Could you check a few things on this drawing? It's one solid part, dimensions in mm from its lowest x, y, z. A direction names the side the tool comes from. Coordinates: 2 decimals unless noted, no trailing zeros. Write each loop counter-clockwise with the first axis right and the second up, starting at its lowest first coordinate (ties: lowest second). Pieces come first, ordered by that corner, then holes.
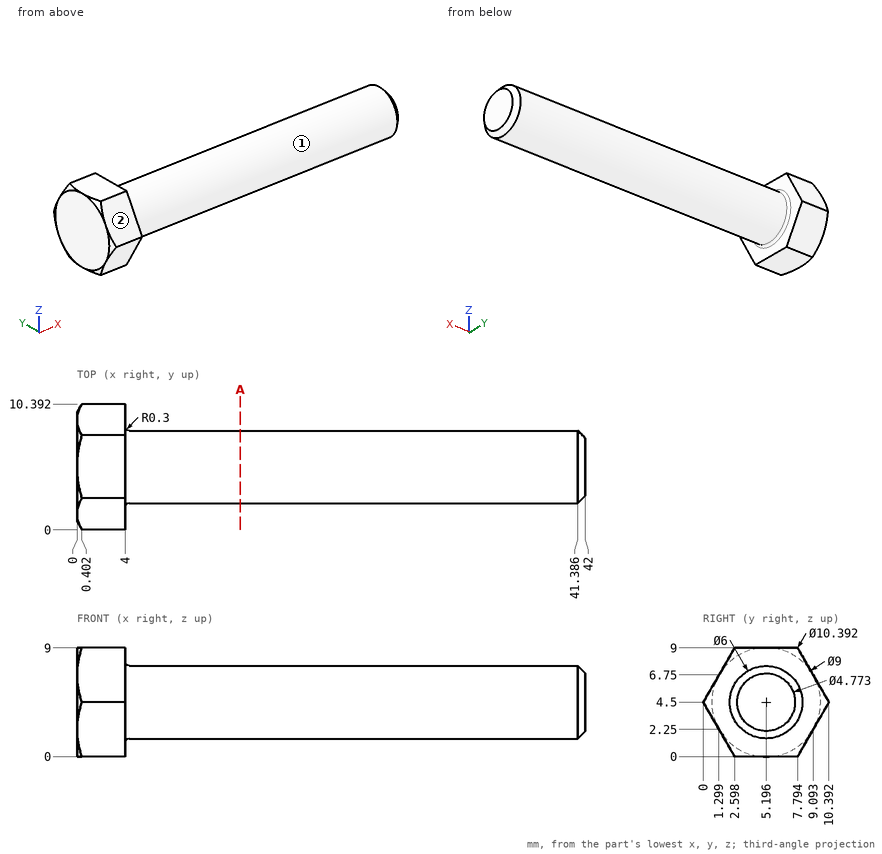
1) Will these pins go through, and if not, where does the flat tip stop? pin 1 (3 mm diameter, centred on x = 35.5, y = 2.5, fed in from +Z); pin 2 (3 mm diameter, centred on x = 23, y = 2.5, fed in from -Z); pin 3 (1 mm diameter, centred on y = 1, z = 4, fed in from +X); pin 4 (1 mm diameter, centred on y = 4.5, z = 3, fed in from -X).
Values follow:
pin 1: stops at z = 7.25
pin 2: stops at z = 1.75
pin 3: stops at x = 4
pin 4: stops at x = 0
2) On a 3-axis mill with a long thin cutter (end or side, diameter ignored), from which of +Z, -Z, +X, -X, +Y, -Y can I reach the whole of each face in a straight line? I mean the marked faces 1 and 2. Say none if no direction works.
Values follow:
face 1: +X
face 2: +Z, +X, -X, -Y
3) I need wall thicknesses on probe 1 along X at (y, z) = (6, 7.75); probe 2 along Z at (x, y) = (29.5, 5.25); probe 3 along Z at (x, y) = (40.5, 7.5). Which ranges of each line are inside material? Lowest first, please.
Values follow:
probe 1: x = 0 to 4
probe 2: z = 1.5 to 7.5
probe 3: z = 2.58 to 6.42
4) Imagine slicing it at A-A on x = 13.5. Please give me the cut outline in (y, z).
Values follow:
outline: circle Ø6 at (5.2, 4.5)
